The model under review builds one solid part; all positions refer to its coordinate system, in mm. Give positions to 0.01 mm unless a question says otherwise; leave off trailing zeros. Write each loop counter-clockwise with the first axis right and the second up, starting at its lowest first coordinate (ties: lowest second). Pieces come first, ordered by that corner, then holes. Notation, with made-up numbers: (16, 83.5) - (58, 83.5) arc R11 cw to (58, 99.5) - close; hole circle Ø4 at (-29.75, -1). An arc over 180 degrees is marked (long way). Write item = value, one per line.
```python
from build123d import *

# Parameters (mm, degrees)
F0_W     = 180
F0_H     = 100
F1_DEPTH = 4
F2_R     = 6
F3_R     = 6
F4_DEPTH = 100


with BuildPart() as f1:
    # F0 (on Front) → F1 (new body)
    with BuildSketch(Plane.XZ):
        with Locations((90, 50)):
            Rectangle(F0_W, F0_H)
    extrude(amount=F1_DEPTH)

    # F2 (on Front) + F3 (on face) → F4 (cut)
    with BuildSketch(Plane.XZ):
        with Locations((25, 80)):
            Circle(F2_R)
    with BuildSketch(Plane(origin=(0, 0, 0), x_dir=(-1, 0, 0), z_dir=(0, 1, 0))):
        with Locations((-155, 20)):
            Circle(F3_R)
        with Locations((-155, 80)):
            Circle(F3_R)
        with Locations((-25, 20)):
            Circle(F3_R)
        with Locations((-90, 80)):
            Circle(F3_R)
        with Locations((-90, 20)):
            Circle(F3_R)
    extrude(amount=F4_DEPTH, dir=(0, -1, 0), mode=Mode.SUBTRACT)


solid = f1.part
```
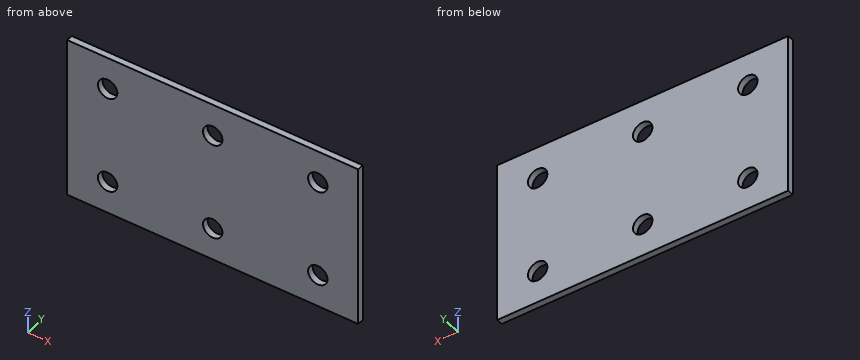
1. Take a section at A-A on y = -1.8. Give the boundary of the cut face in (x, z).
Findings below:
outline = (0, 0) - (180, 0) - (180, 100) - (0, 100) - close; hole circle Ø12 at (25, 20); hole circle Ø12 at (25, 80); hole circle Ø12 at (90, 20); hole circle Ø12 at (90, 80); hole circle Ø12 at (155, 20); hole circle Ø12 at (155, 80)
2. For line 1 (Z direction, x = 90, y = -0.8); line 2 (X direction, y = -1.9, z = 17); line 3 (Z direction, x = 95, y = -2.1), list the stretches that pass through material, from the lowest coordinate up. Write a range as from..to.
Findings below:
line_1 = 0..14, 26..74, 86..100
line_2 = 0..19.8, 30.2..84.8, 95.2..149.8, 160.2..180
line_3 = 0..16.68, 23.32..76.68, 83.32..100
3. Take a section at B-B on x = 25. Give the boundary of the cut face in (y, z).
Findings below:
outline = (-4, 0) - (0, 0) - (0, 14) - (-4, 14) - close; (-4, 26) - (0, 26) - (0, 74) - (-4, 74) - close; (-4, 86) - (0, 86) - (0, 100) - (-4, 100) - close
4. Insertion check: P1, Ø7, axis at x = 155, z = 80, coming from the +Y side. The pin has a flat end and moves straight along its axis. Give the tip position at first contact, or say it passes through.
Findings below:
P1 = through
5. Take a section at C-C on z = 20. Give the boundary of the cut face in (x, y), and give its area (3 significant figures).
Findings below:
outline = (0, -4) - (19, -4) - (19, 0) - (0, 0) - close; (31, -4) - (84, -4) - (84, 0) - (31, 0) - close; (96, -4) - (149, -4) - (149, 0) - (96, 0) - close; (161, -4) - (180, -4) - (180, 0) - (161, 0) - close
area = 576 mm²
